Read the model definition and answer for the solid it produces. Units are mm, in the model's axes. Coordinates: 2 decimals unless noted, no trailing zeros. Loops run counter-clockwise (first coordinate to the right, second up) from the corner with the lowest first, then second, coordinate; pieces in that order, holes last. Notation, with made-up numbers: (26, -39.75) - (59, -39.75) arc R34 cw to (59, -0.75) - close; hole circle Ø11 at (39, 52.5). An arc over 180 degrees is marked (long way). Use CSV: the item, a comma, the result in double quotes.
```python
from build123d import *

# Parameters (mm, degrees)
BOSS_EXTRUDE1_DEPTH = 6.35
FILLET1_R           = 1.905


with BuildPart() as part:
    # Sketch1 → Boss-Extrude1 (new body)
    with BuildSketch(Plane(origin=(0, 0, 0), x_dir=(1, 0, 0), z_dir=(0, 1, 0))):
        with BuildLine():
            Line((-44.45, 68.072), (44.45, 68.072))
            Line((44.45, 68.072), (44.45, 50.927))
            Line((44.45, 50.927), (31.510734202, 37.553030691))
            ThreePointArc((31.510734202, 37.553030691), (0, 49.022), (-31.510734202, 37.553030691))
            Line((-31.510734202, 37.553030691), (-44.45, 50.927))
            Line((-44.45, 50.927), (-44.45, 68.072))
        make_face()
    extrude(amount=BOSS_EXTRUDE1_DEPTH)

    # Fillet1
    fillet1_edges = [part.edges().sort_by_distance(p)[0] for p in [
        (31.510734202, 3.175, -37.553030691),
        (-31.510734202, 3.175, -37.553030691),
        (0, 6.35, -49.022),
        (0, 0, -49.022),
    ]]
    fillet(fillet1_edges, radius=FILLET1_R)


solid = part.part
```
Q1. The part is cut by section B-B on x = 39.5. Determine the outline of the cut face in (y, z).
Reported:
outline,"(0, -68.07) - (6.35, -68.07) - (6.35, -45.81) - (0, -45.81) - close"
Q2. Find the intervals of material crossed by probe 1 along Z at (x, y) = (-33.5, 4.25); probe 2 along Z at (x, y) = (-39, 6.25); probe 3 along X at (y, z) = (2, -40), in increasing order. Write a range as [from, to].
Reported:
probe 1,"z = [-68.07, -39.61]"
probe 2,"z = [-68.07, -45.29]"
probe 3,"x = [-33.88, -28.34], [28.34, 33.88]"
Q3. The part is cut by section A-A on y = 3.5. Determine the outline of the cut face in (x, z) (3 decimals), and give its area (3 significant figures).
Reported:
outline,"(-44.45, -68.072) - (44.45, -68.072) - (44.45, -50.927) - (32.723, -38.806) arc R1.905 ccw to (30.181, -38.63) arc R49.022 cw to (-30.181, -38.63) arc R1.905 ccw to (-32.723, -38.806) - (-44.45, -50.927) - close"
area,"2,040 mm²"
Q4. For a pull along X with two mould halves and no side action, classify faces 1 (the face through (-31.77, 3.22, -38.27)), 2 (the face through (1, 0, -57)), 3 (the face through (38.67, 3.13, -44.95)) as +X half, -X half, draft (parallel to the pull), parting line (faces both ways), or undercut.
Reported:
face 1,"undercut"
face 2,"draft"
face 3,"+X half"
